Work out the finished part from the listing and answer in its coordinate system (mm). Face numbers are marked on the shaded views. A direction names the side the tool comes from. Give positions to 0.01 mm unless a question says otherwise; leave off trailing zeros. Order: outer loops, then holes, each group sorted by start corner. A loop starts at its lowest first (then second) coordinate and runs counter-clockwise, first axis right, second up. Notation, with made-up numbers: (-28, -17) - (16, -17) arc R18 cw to (16, -4) - close; hole circle Ø11 at (41.25, 86). An arc over 180 degrees is marked (long way). Write each question's results on one line, items separated by ' | '.
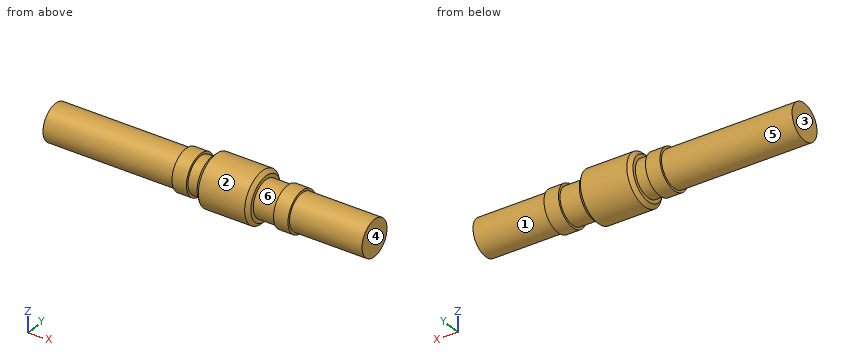
from build123d import *

# Parameters (mm, degrees)
CROQUIS1_R              = 35
SALIENTE_EXTRUIR1_DEPTH = 37
CHAFL_N1_SIZE           = 5
CROQUIS2_R              = 25
SALIENTE_EXTRUIR2_DEPTH = 16
CROQUIS3_R              = 28.1
SALIENTE_EXTRUIR3_DEPTH = 120
SALIENTE_EXTRUIR4_START = 30
CROQUIS4_R              = 25
SALIENTE_EXTRUIR4_DEPTH = 30
SALIENTE_EXTRUIR5_START = 120
CROQUIS5_R              = 28.1
SALIENTE_EXTRUIR5_DEPTH = 120
CORTAR_EXTRUIR1_START   = -100
CROQUIS6_R              = 28.1
CROQUIS6_R_2            = 25
CORTAR_EXTRUIR1_DEPTH   = 100
CROQUIS8_R              = 28.1
CROQUIS8_R_2            = 25
CORTAR_EXTRUIR2_DEPTH   = 100
CROQUIS9_R              = 25
SALIENTE_EXTRUIR6_DEPTH = 80


with BuildPart() as part:
    # Croquis1 → Saliente-Extruir1 (new, symmetric)
    with BuildSketch(Plane(origin=(0, 0, 0), x_dir=(0, 0, -1), z_dir=(1, 0, 0))):
        Circle(CROQUIS1_R)
    extrude(amount=SALIENTE_EXTRUIR1_DEPTH, both=True)

    # Chaflán1
    chafl_n1_edges = [part.edges().sort_by_distance(p)[0] for p in [
        (-37, 0, 35),
        (37, 0, 35),
    ]]
    chamfer(chafl_n1_edges, length=CHAFL_N1_SIZE)

    # Croquis2 → Saliente-Extruir2 (add)
    with BuildSketch(Plane.ZY.offset(37)):
        Circle(CROQUIS2_R)
    extrude(amount=SALIENTE_EXTRUIR2_DEPTH)

    # Croquis3 → Saliente-Extruir3 (add)
    with BuildSketch(Plane.ZY.offset(53)):
        Circle(CROQUIS3_R)
    extrude(amount=SALIENTE_EXTRUIR3_DEPTH)

    # Croquis4 → Saliente-Extruir4 (add)
    with BuildSketch(Plane(origin=(37, 0, 0), x_dir=(0, 0, -1), z_dir=(1, 0, 0)).offset(SALIENTE_EXTRUIR4_START)):
        with Locations(Location((0, 0, 0), (0, 0, 180))):
            Circle(CROQUIS4_R)
    extrude(amount=-SALIENTE_EXTRUIR4_DEPTH)

    # Croquis5 → Saliente-Extruir5 (add)
    with BuildSketch(Plane(origin=(67, 0, 0), x_dir=(0, 0, -1), z_dir=(1, 0, 0)).offset(SALIENTE_EXTRUIR5_START)):
        with Locations(Location((0, 0, 0), (0, 0, 180))):
            Circle(CROQUIS5_R)
    extrude(amount=-SALIENTE_EXTRUIR5_DEPTH)

    # Croquis6 → Cortar-Extruir1 (cut)
    with BuildSketch(Plane.ZY.offset(173).offset(CORTAR_EXTRUIR1_START)):
        Circle(CROQUIS6_R)
        Circle(CROQUIS6_R_2, mode=Mode.SUBTRACT)
    extrude(amount=CORTAR_EXTRUIR1_DEPTH, mode=Mode.SUBTRACT)

    # Croquis8 → Cortar-Extruir2 (cut)
    with BuildSketch(Plane(origin=(187, 0, 0), x_dir=(0, 0, -1), z_dir=(1, 0, 0))):
        with Locations(Location((0, 0, 0), (0, 0, 180))):
            Circle(CROQUIS8_R)
        with Locations(Location((0, 0, 0), (0, 0, 180))):
            Circle(CROQUIS8_R_2, mode=Mode.SUBTRACT)
    extrude(amount=-CORTAR_EXTRUIR2_DEPTH, mode=Mode.SUBTRACT)

    # Croquis9 → Saliente-Extruir6 (add)
    with BuildSketch(Plane.ZY.offset(173)):
        Circle(CROQUIS9_R)
    extrude(amount=SALIENTE_EXTRUIR6_DEPTH)


solid = part.part
1. Determine the mould class of the marked faces 3, 4, 5 and 6 for opening direction X: +X half, -X half, draft (parallel to the pull), parting line (faces both ways), or undercut.
Answer list:
face 3: -X half | face 4: +X half | face 5: draft | face 6: undercut
2. A cutting plane is placed at C-C, the plane x = 148.5. Write down the section's boundary in (y, z).
Answer list:
outline: circle Ø50 at (0, 0)
3. Straight lines are drawn through the part: line 1 (X direction, y = -26, z = 6); line 2 (Y direction, x = 17, z = -2.5); line 3 (X direction, y = -8, z = 27). For each, find the intervals that lie inside material, in ascending order. Write a range as [from, to].
Answer list:
line 1: [-73, -53], [-37, 37], [67, 87] | line 2: [-34.91, 34.91] | line 3: [-37, 37]
4. Given P1, Ø4, axis at x = 32, z = 4, coming from the +Y side; P2, Ø12, axis at x = -54, z = -1.5, coming from the -Y side; P3, Ø3, axis at y = -27, z = -7, coming from the -X side, each flat-ended and moving along its own axis, determine where each tip first touches the part or whether it passes through.
Answer list:
P1: y = 34.94 | P2: y = -28.1 | P3: x = -73
5. A cutting plane is placed at D-D, the plane x = 0. Write down the section's boundary in (y, z), then the cut area to 3 significant figures.
Answer list:
outline: circle Ø70 at (0, 0) | area: 3,850 mm^2
6. A tool of negligible diameter and unlimited length cuts with its end or side. For the marked faces 1 and 2, from which of +Z, -Z, +X, -X, +Y, -Y can it reach the whole face along a straight path? Write none if from no direction.
Answer list:
face 1: +X | face 2: +X, -X
